from build123d import *

# Parameters (mm, degrees)
BOSS_EXTRUDE3_DEPTH     = 10
SKETCH3_R               = 10
BOSS_EXTRUDE4_DEPTH     = 8
SKETCH7_R               = 1.7
CUT_EXTRUDE2_DEPTH      = 2
CUT_EXTRUDE2_DEPTH_BACK = 35.997647024
SKETCH8_W               = 6
SKETCH8_H               = 3
CUT_EXTRUDE3_DEPTH      = 6.8


with BuildPart() as part:
    # Sketch1 → Boss-Extrude3 (new body)
    with BuildSketch(Plane.XY):
        Polygon((16.278404236, 26.406692505), (15.44379425, 27.927993774), (15.101806641, 29.638374329), (15.70716095, 30.097465515), (17.261032104, 29.306182861), (18.501731873, 28.092857361), (19.338500977, 28.410926819), (19.458862305, 30.141960144), (20.095863342, 31.765708923), (20.85332489, 31.824638367), (21.732727051, 30.318885803), (22.120491028, 28.62739563), (22.996398926, 28.442581177), (24.03351593, 29.833747864), (25.447257996, 30.85533905), (26.116333008, 30.495407104), (26.042068481, 28.753242493), (25.453788757, 27.120628357), (26.09072876, 26.491607666), (27.715324402, 27.101219177), (29.456954956, 27.196311951), (29.82522583, 26.531791687), (28.820861816, 25.106338501), (27.443313599, 24.050941467), (27.639060974, 23.17742157), (29.335342407, 22.811935425), (30.851913452, 21.950332642), (30.802444458, 21.192199707), (29.18686676, 20.53603363), (27.45741272, 20.392944336), (27.14982605, 19.552253723), (28.379226685, 18.327713013), (29.189224243, 16.782974243), (28.737739563, 16.171928406), (27.023872375, 16.493377686), (25.491607666, 17.308013916), (24.778335571, 16.767074585), (25.150535583, 15.072257996), (24.996803284, 13.334815979), (24.286636353, 13.064868927), (23.018630981, 14.261878967), (22.170021057, 15.775596619), (21.277534485, 15.70615387), (20.674362183, 14.079162598), (19.605697632, 12.700645447), (18.862319946, 12.857494354), (18.442756653, 14.550018311), (18.54724884, 16.282234192), (17.758888245, 16.706329346), (16.37184906, 15.663711548), (14.727554321, 15.081794739), (14.186981201, 15.615646362), (14.749069214, 17.266319275), (15.773483276, 18.667060852), (15.339553833, 19.450050354), (13.609024048, 19.32283783), (11.911148071, 19.722267151), (11.745010376, 20.463630676), (13.110290527, 21.548377991), (14.729377747, 22.172920227), (14.787651062, 23.066207886), (13.263061523, 23.89478302), (12.05065918, 25.148750305), (12.311706543, 25.862243652), (14.046714783, 26.03666687), (15.746429443, 25.686714172), align=None)
        with BuildLine():
            Line((19.728870468, 19.947937012), (22.713832779, 19.947937012))
            ThreePointArc((22.713832779, 19.947937012), (21.221351624, 24.897937012), (19.728870468, 19.947937012))
        make_face(mode=Mode.SUBTRACT)
    extrude(amount=BOSS_EXTRUDE3_DEPTH)

    # Sketch3 → Boss-Extrude4 (add)
    with BuildSketch(Plane(origin=(0, 0, 0), x_dir=(-1, 0, 0), z_dir=(0, 0, -1))):
        with Locations((-21.221351624, 22.197937012)):
            Circle(SKETCH3_R)
        with BuildLine():
            Line((-19.728870468, 19.947937012), (-22.713832779, 19.947937012))
            ThreePointArc((-22.713832779, 19.947937012), (-21.221351624, 24.897937012), (-19.728870468, 19.947937012))
        make_face(mode=Mode.SUBTRACT)
    extrude(amount=BOSS_EXTRUDE4_DEPTH)

    # Sketch7 → Cut-Extrude2 (cut, two sides)
    with BuildSketch(Plane(origin=(0, 19.947937012, 0), x_dir=(1, 0, 0), z_dir=(0, 1, 0))) as cut_extrude2_sk:
        with Locations(Location((21.221351624, 4.6, 0), (0, 0, 90))):
            Circle(SKETCH7_R)
    extrude(amount=CUT_EXTRUDE2_DEPTH, mode=Mode.SUBTRACT)
    extrude(cut_extrude2_sk.sketch, amount=-CUT_EXTRUDE2_DEPTH_BACK, mode=Mode.SUBTRACT)

    # Sketch8 → Cut-Extrude3 (cut)
    with BuildSketch(Plane(origin=(0, 0, -8), x_dir=(-1, 0, 0), z_dir=(0, 0, -1))):
        with Locations((-21.221351624, 17.197937012)):
            Rectangle(SKETCH8_W, SKETCH8_H)
    extrude(amount=-CUT_EXTRUDE3_DEPTH, mode=Mode.SUBTRACT)


solid = part.part
Build history of the part. All positions in model axes, mm. A direction names the side the tool comes from. Coordinates: 2 decimals unless noted, no trailing zeros. Order: outer loops, then holes, each group sorted by start corner. A loop starts at its lowest first (then second) coordinate and runs counter-clockwise, first axis right, second up. Notation, with made-up numbers: (32.5, 73.5) -> (70.5, 73.5) arc R16 cw to (70.5, 84.5) -> close; hole circle Ø4 at (53, 50.25). An arc over 180 degrees is marked (long way). One line per item, written item: value.
(1) Tool access for faces 4 (the flat face through (15.561, 15.377, 4.93)), 5 (the flat face through (13.909, 21.856, 4.93)), 6 (the flat face through (12.77, 19.52, 4.93)): list every direction of +Z, -Z, +X, -X, +Y, -Y with a clear straight run to the whole face (end or side of a thin tool).
Checked values:
face 4: +Z, -Y
face 5: +Z, -X
face 6: +Z, -X, -Y
(2) Probe line 1 (Y direction, x = 20.5, z = -1.25); line 2 (Y direction, x = 28.5, z = 2); line 3 (X direction, y = 13.4, z = -4.6). List the from-to ranges inside material, lowest first. Write a range as [from, to].
Checked values:
line 1: [12.22, 15.7], [18.7, 19.95], [24.8, 32.17]
line 2: [16.22, 18.1], [20.48, 22.99], [24.86, 27.14]
line 3: [16.47, 19.52], [22.92, 25.97]
(3) Slice it at B-B, the plane z = -0.5. List the corners of the cut face in (x, y).
Checked values:
outline: circle Ø20 at (21.22, 22.2); hole (19.73, 19.95) -> (22.71, 19.95) arc R2.7 ccw (long way) to start
(4) Slice it at A-A, the plane z = -4.6. List the corners of the cut face in (x, y).
Checked values:
outline: (18.22, 15.7) -> (18.22, 18.7) -> (19.52, 18.7) -> (19.52, 20.1) arc R2.7 cw (long way) to (22.92, 20.1) -> (22.92, 18.7) -> (24.22, 18.7) -> (24.22, 15.7) -> (22.92, 15.7) -> (22.92, 12.34) arc R10 ccw (long way) to (19.52, 12.34) -> (19.52, 15.7) -> close
(5) Mould opens along Z. For faces 1 (the flat face through (23, 29, 0)), 2 (the cylindrical face through (21.15, 19.41, -2.9)), 3 (the flat face through (20.15, 13.4, 4.93)) say: pulls with the +Z half, pulls with the -Z half, needs draft (parallel to the pull), parting line crosses it, or undercut.
Checked values:
face 1: pulls with the +Z half
face 2: undercut
face 3: needs draft
(6) Drop flat-ended pins along their axis: pin 1 Ø8 at (y, z) = (27.5, 2) entering from +X; pin 2 Ø5 at (y, z) = (27, 6.5) entering from -X; pin 3 Ø2.5 at (y, z) = (17.5, -5) entering from -X. Give the stop position or say it passes through.
Checked values:
pin 1: x = 31.05
pin 2: x = 12.05
pin 3: x = 11.83
